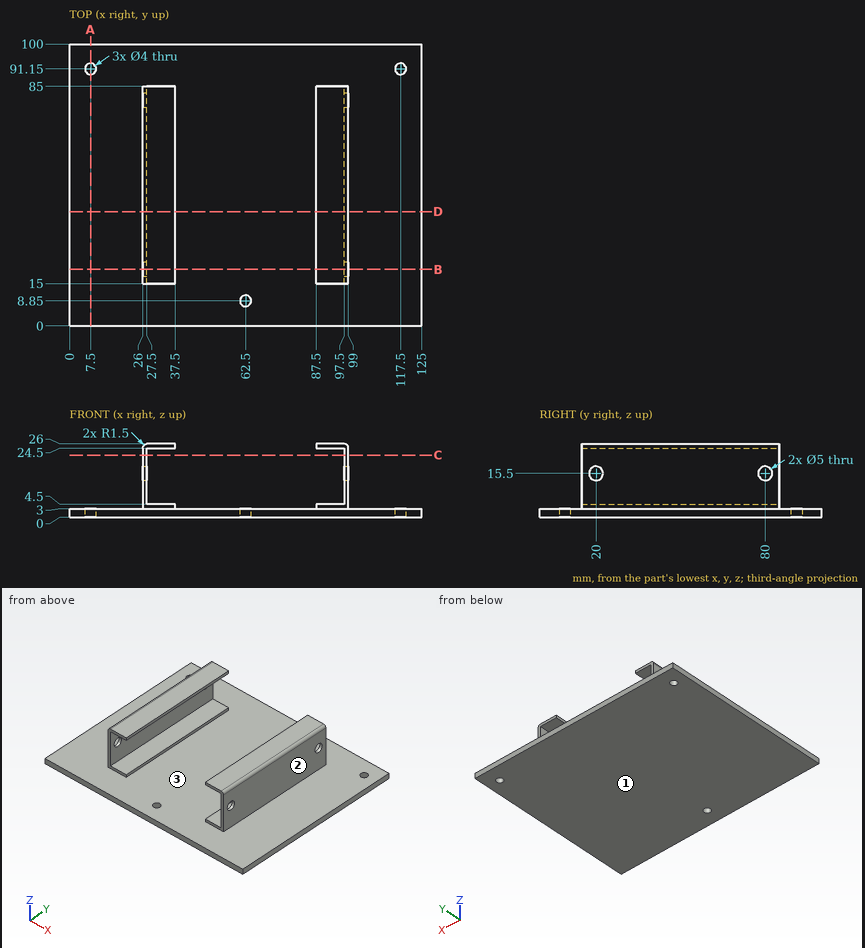
Could you check a few things on this drawing? It's one solid part, dimensions in mm from its lowest x, y, z. Coordinates: 2 decimals unless noted, no trailing zeros. Loops run counter-clockwise (first coordinate to the right, second up) from the corner with the lowest first, then second, coordinate; pieces in that order, holes last. Notation, with made-up numbers: (47, 9.25) - (91, 9.25) arc R29 ccw to (91, 35.25) - close; hole circle Ø5 at (40.25, 78.5). An arc over 180 degrees is marked (long way). Answer as a JSON object with one key per item and string values. Group by question number.
Item 1: If we section it at C-C (z = 22): List the corners of the cut face in (x, y) for me, plus the area to 3 significant figures.
Item 2: If we section it at B-B (y = 20): State how many separate pieces and enclosed holes the cut face has, plus the area to 3 significant figures.
Item 3: If we section it at D-D (y = 40.5): List the corners of the cut face in (x, z) for me, plus the area to 3 significant figures.
Item 4: If I drill on L1, parallel to Z at x = 32, y = 58; L2, parallel to X at y = 91.15, z = 2.25; L3, parallel to X at y = 29.5, z = 10, over which ranges is the centre line in solid material (lowest first)? Write a range as from..to.
Item 5: If we mould it in two halves opening along X, with no side actions, what happens to the marked faces 1, 2 and 3? For each: released by +X, released by -X, zero draft, split by the parting line, or undercut.
Item 6: If we section it at A-A (x = 7.5): List the corners of the cut face in (y, z) for me, plus the area to 3 significant figures.
Item 7: For pin 1 (6 mm diameter, centred on y = 41, z = 17, fed in from +X); pin 2 (9 mm diameter, centred on x = 90.5, z = 9.5, fed in from -Y); pin 3 (12 mm diameter, centred on x = 99.5, z = 10.5, fed in from +Y); pin 4 (4 mm diameter, centred on x = 43.5, y = 68.5, fed in from +Z), each with a flat end and sliding along its axis, tell me the tip position at first contact or that it passes through.
Returned:
{
 "1": {"outline": "(26, 15) - (27.5, 15) - (27.5, 85) - (26, 85) - close; (97.5, 15) - (99, 15) - (99, 85) - (97.5, 85) - close", "area": "210 mm²"},
 "2": {"separate pieces": "3", "enclosed holes": "0", "area": "488 mm²"},
 "3": {"outline": "(0, 0) - (125, 0) - (125, 3) - (99, 3) - (99, 24.5) arc R1.5 ccw to (97.5, 26) - (87.5, 26) - (87.5, 24.5) - (97.5, 24.5) - (97.5, 4.5) - (87.5, 4.5) - (87.5, 3) - (37.5, 3) - (37.5, 4.5) - (27.5, 4.5) - (27.5, 24.5) - (37.5, 24.5) - (37.5, 26) - (27.5, 26) arc R1.5 ccw to (26, 24.5) - (26, 3) - (0, 3) - close", "area": "503 mm²"},
 "4": {"L1": "z = 0..4.5, 24.5..26", "L2": "x = 0..5.5, 9.5..115.5, 119.5..125", "L3": "x = 26..27.5, 97.5..99"},
 "5": {"face 1": "zero draft", "face 2": "released by +X", "face 3": "undercut"},
 "6": {"outline": "(0, 0) - (89.15, 0) - (89.15, 3) - (0, 3) - close; (93.15, 0) - (100, 0) - (100, 3) - (93.15, 3) - close", "area": "288 mm²"},
 "7": {"pin 1": "stops at x = 99", "pin 2": "passes through", "pin 3": "stops at y = 85", "pin 4": "stops at z = 3"}
}
